Could you check a few things on this model? Use its own coordinates, in mm. A direction names the side the tool comes from. Give positions to 0.01 mm unless a question says otherwise; leave off trailing zeros. Loops run counter-clockwise (first coordinate to the right, second up) from the corner with the lowest first, then second, coordinate; pieces in that order, holes last. Notation, with made-up numbers: (87.5, 79) - (111.5, 79) arc R16 ccw to (111.5, 93) - close; hole circle Ø10 at (38.25, 58.25). An arc over 180 degrees is marked (long way). Answer in a Markdown table with one row per item. Add a question column.
```python
from build123d import *

# Parameters (mm, degrees)
SKETCH2_W          = 2
SKETCH2_H          = 5
CUT_EXTRUDE1_DEPTH = 1
SKETCH4_W          = 2
SKETCH4_H          = 3
CUT_EXTRUDE2_DEPTH = 1


with BuildPart() as part:
    # Sketch1 → Revolve1 (revolve)
    with BuildSketch(Plane.XY, mode=Mode.PRIVATE) as revolve1_sk:
        Polygon((0, 0), (0, -1.5), (10, -1.5), (10, -2.5), (12, -2.5), (12, 0), align=None)
    revolve(revolve1_sk.sketch.rotate(Axis((12, 0, 0), (-1, 0, 0)), 270), axis=Axis((12, 0, 0), (-1, 0, 0)))

    # Sketch2 → Cut-Extrude1 (cut)
    with BuildSketch(Plane(origin=(0, 3, 0), x_dir=(1, 0, 0), z_dir=(0, 1, 0))):
        with Locations((11, 0)):
            Rectangle(SKETCH2_W, SKETCH2_H)
    extrude(amount=-CUT_EXTRUDE1_DEPTH, mode=Mode.SUBTRACT)

    # Sketch4 → Cut-Extrude2 (cut)
    with BuildSketch(Plane(origin=(0, -3, 0), x_dir=(1, 0, 0), z_dir=(0, 1, 0))):
        with Locations((11, 0)):
            Rectangle(SKETCH4_W, SKETCH4_H)
    extrude(amount=CUT_EXTRUDE2_DEPTH, mode=Mode.SUBTRACT)


solid = part.part
```
(1) For pin 1 Ø2 at (x, z) = (1.5, 0.5) entering from +Y, with a flat end and sliding along its axis, tell me the tip position at first contact or that it passes through.
(2) I want a section at A-A on z = 0. Please give me the cut outline in (x, y).
(3) On a 3-axis mill with a long thin cutter (end or side, diameter ignored), from which of +Z, -Z, +X, -X, +Y, -Y can I reach the whole of each face in a straight line? I mean faces 1 (the cylindrical face through (11, 0, 2.5)), 2 (the cylindrical face through (5.07, -0.45, -1.43)). Say none if no direction works.
(4) I want a section at D-D on z = -2.1. Please give me the cut outline in (x, y), then the cut area to 3 significant figures.
(5) Please list where these lines run through material, in increasing order: line 1 (X direction, y = 1.7, z = -0.35); line 2 (Y direction, x = 10.75, z = 2); line 3 (Y direction, x = 10.5, z = -1.95).
(6) I want a section at B-B on y = 0. Please give me the cut outline in (x, z), then the cut area to 3 significant figures.
(7) I want a section at C-C on x = 7.75. Please give me the cut outline in (y, z), then the cut area to 3 significant figures.
Reported:
| question | item | result |
|---|---|---|
| 1 | pin 1 | y = 1.5 |
| 2 | outline | (0, -1.5) - (10, -1.5) - (10, -2) - (12, -2) - (12, 2) - (10, 2) - (10, 1.5) - (0, 1.5) - close |
| 3 | face 1 | +Z, +X, -X |
| 3 | face 2 | -X |
| 4 | outline | (10, -1.36) - (12, -1.36) - (12, 1.36) - (10, 1.36) - close |
| 4 | area | 5.43 mm² |
| 5 | line 1 | 10 to 12 |
| 5 | line 2 | -1.5 to 1.5 |
| 5 | line 3 | -1.56 to 1.56 |
| 6 | outline | (0, -1.5) - (10, -1.5) - (10, -2.5) - (12, -2.5) - (12, 2.5) - (10, 2.5) - (10, 1.5) - (0, 1.5) - close |
| 6 | area | 40.0 mm² |
| 7 | outline | circle Ø3 at (0, 0) |
| 7 | area | 7.07 mm² |
